Could you check a few things on this drawing? It's one solid part, dimensions in mm from its lowest x, y, z. A direction names the side the tool comes from. Coordinates: 2 decimals unless noted, no trailing zeros. Loops run counter-clockwise (first coordinate to the right, second up) from the corner with the lowest first, then second, coordinate; pieces in that order, holes last. Notation, with made-up numbers: M 76.5,-33 L 107.5,-33 A21 cw 107.5,-3 Z; hole C 55.25,-28 d9. An arc over 180 degrees is marked long. Answer as a JSON object with one key per item and string values. Group by question number.
Item 1: Suppose I cut it at D-D (y = 36). Write out the boundary of the cut face in (x, z).
Item 2: We'd pull the mould along X, two halves only. Please class the marked faces 4, 5 and 6: +X half, -X half, draft (parallel to the pull), parting line (faces both ways), or undercut.
Item 3: Suppose I cut it at A-A (y = 11.5). Write out the boundary of the cut face in (x, z).
Item 4: Suppose I cut it at C-C (z = 19.05). Write out the boundary of the cut face in (x, y).
Item 5: Suppose I cut it at B-B (x = 7.62). Write out the boundary of the cut face in (y, z).
Item 6: If I drill on line 1 (Z direction, x = 7, y = 3); line 2 (X direction, y = 13.75, z = 82.55) (1 decimal); line 3 (Y direction, x = 7.5, z = 46), over which ranges is the centre line in solid material (lowest first)?
Item 7: Which directions (+Z, -Z, +X, -X, +Y, -Y) give clear straight access to the entire face, cutting with the end or side of a thin tool? Please do the marked faces 1, 2 and 3.
Item 8: I'm going to push flat-ended pins straight in: pin 1 Ø4 at (x, z) = (6, 75.5) entering from +Y; pin 2 Ø6 at (y, z) = (40, 15.5) entering from -X (1 decimal); pin 3 Ø1.5 at (y, z) = (29.5, 85) entering from +X. Where does each tip first touch, or does it pass through?
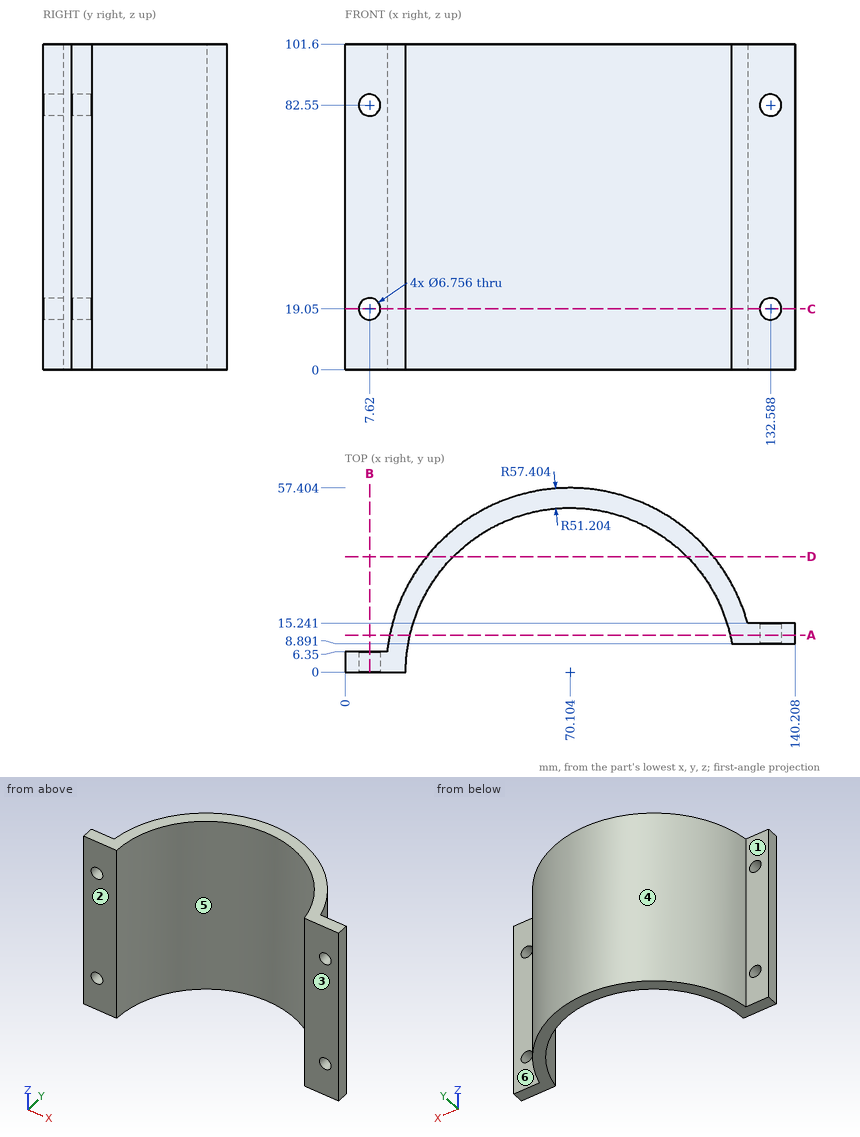
From the geometry:
{
 "1": {"outline": "M 25.39,0 L 33.69,0 L 33.69,101.6 L 25.39,101.6 Z; M 106.52,0 L 114.82,0 L 114.82,101.6 L 106.52,101.6 Z"},
 "2": {"face 4": "parting line", "face 5": "undercut", "face 6": "draft"},
 "3": {"outline": "M 13.86,0 L 20.21,0 L 20.21,101.6 L 13.86,101.6 Z; M 120,0 L 140.21,0 L 140.21,101.6 L 120,101.6 Z; hole C 132.59,19.05 d6.76; hole C 132.59,82.55 d6.76"},
 "4": {"outline": "M 0,0 L 4.24,0 L 4.24,6.35 L 0,6.35 Z; M 11,0 L 18.9,0 A51.2 cw 120.53,8.89 L 129.21,8.89 L 129.21,15.24 L 125.45,15.24 A57.4 ccw 13.05,6.35 L 11,6.35 Z; M 135.97,8.89 L 140.21,8.89 L 140.21,15.24 L 135.97,15.24 Z"},
 "5": {"outline": "M 0,0 L 6.35,0 L 6.35,15.67 L 0,15.67 Z; M 0,22.43 L 6.35,22.43 L 6.35,79.17 L 0,79.17 Z; M 0,85.93 L 6.35,85.93 L 6.35,101.6 L 0,101.6 Z"},
 "6": {"line 1": "0 to 15.73, 22.37 to 79.23, 85.87 to 101.6", "line 2": "14.4 to 20.8, 119.4 to 129.2, 136 to 140.2", "line 3": "0 to 6.35"},
 "7": {"face 1": "+Z, -Z, -X, +Y", "face 2": "+Z, -Z, +X, -X, -Y", "face 3": "+Z, -Z, +X, -Y"},
 "8": {"pin 1": "y = 6.35", "pin 2": "x = 26.2", "pin 3": "x = 119.79"}
}
